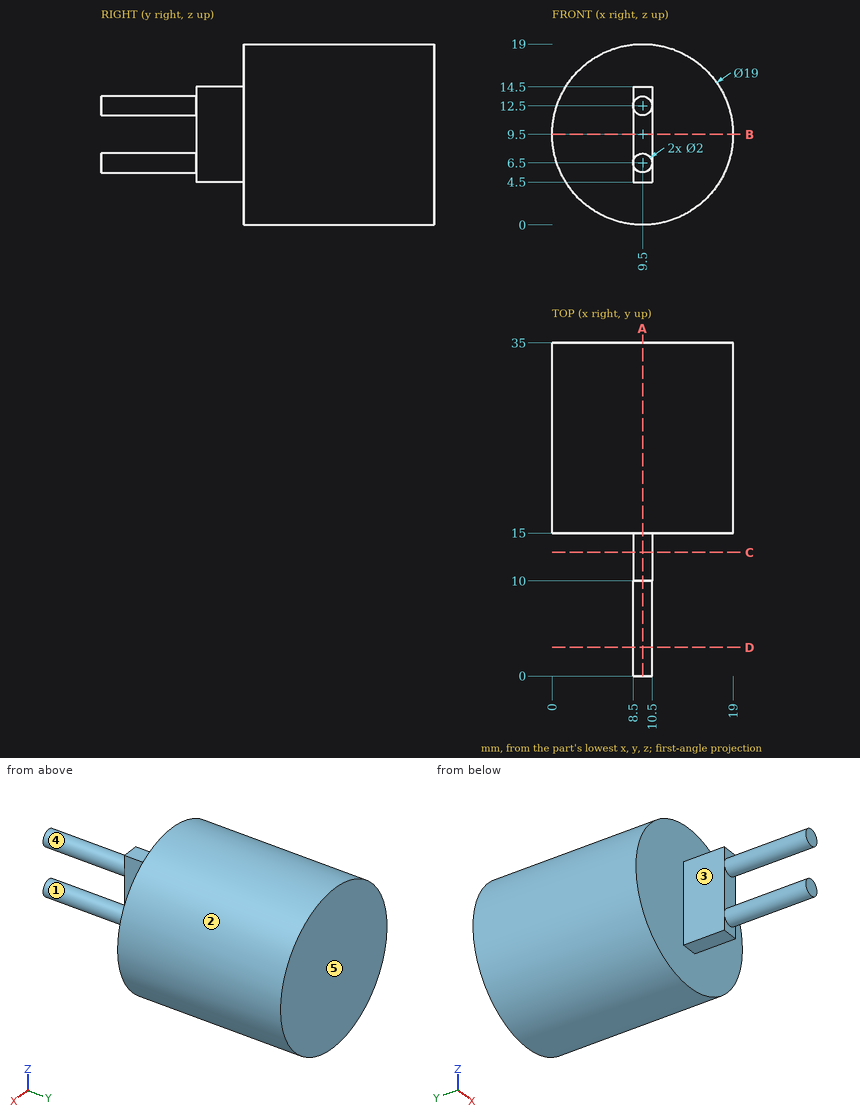
Job drawing, mm, ordinate dimensions from the low corner. One solid piece. A direction names the side the tool comes from. Round coordinates to 2 decimals unless told otherwise and drop trailing zeros. Loops run counter-clockwise (first coordinate to the right, second up) from the corner with the lowest first, then second, coordinate; pieces in that order, holes last.
(1) Two-plate mould, pull along Z, no slides. Class the marked faces 1, 2 and 3: +Z half, -Z half, draft (parallel to the pull), parting line (faces both ways), or undercut.
(2) Cut at D-D (y = 3). Give the cut face in (x, z).
(3) Cut at C-C (y = 13). Give the cut face in (x, z), plus the area to 3 significant figures.
(4) Drop flat-ended pins along their axis: pin 1 (0.6 mm diameter, centred on x = 9.5, y = 13.5, fed in from +Z); pin 2 (2.5 mm diameter, centred on y = 13.5, z = 9, fed in from +X); pin 3 (2 mm diameter, centred on x = 3, y = 31.5, fed in from +Z). Give the stop position or say it passes through.
(5) Cut at A-A (x = 9.5). Give the cut face in (y, z).
(6) Which spindle directions (+Z, -Z, +X, -X, +Y, -Y) get a long thin tool onto all of the face, cutting with end or side? Do the marked faces 4 and 5. Say none if no direction does.
(7) Wall check: line 1 along Y through (x, z) = (8.25, 8.5); line 2 along X through (y, z) = (14.5, 6); line 3 along X through (y, z) = (3.5, 13). Give the ranges that are in metal, low to high.
(8) Cut at B-B (z = 9.5). Give the cut face in (x, y).
Findings below:
1. face 1: undercut
1. face 2: parting line
1. face 3: draft
2. outline: circle Ø2 at (9.5, 6.5); circle Ø2 at (9.5, 12.5)
3. outline: (8.5, 4.5) - (10.5, 4.5) - (10.5, 14.5) - (8.5, 14.5) - close
3. area: 20.0 mm2
4. pin 1: stops at z = 14.5
4. pin 2: stops at x = 10.5
4. pin 3: stops at z = 17.25
5. outline: (0, 5.5) - (10, 5.5) - (10, 4.5) - (15, 4.5) - (15, 0) - (35, 0) - (35, 19) - (15, 19) - (15, 14.5) - (10, 14.5) - (10, 13.5) - (0, 13.5) - (0, 11.5) - (10, 11.5) - (10, 7.5) - (0, 7.5) - close
6. face 4: -Y
6. face 5: +Z, -Z, +X, -X, +Y
7. line 1: y = 15 to 35
7. line 2: x = 8.5 to 10.5
7. line 3: x = 8.63 to 10.37
8. outline: (0, 15) - (8.5, 15) - (8.5, 10) - (10.5, 10) - (10.5, 15) - (19, 15) - (19, 35) - (0, 35) - close
